Can you work these out from the model? Positions are in its coordinate system, mm. Face numbers are marked on the shaded views. A direction names the side the tool comes from. Round coordinates to 2 decimals unless told otherwise and drop trailing zeros. Order: outer loops, then holes, each group sorted by start corner. A loop starts at its lowest first (then second) coordinate and runs counter-clockwise, first axis right, second up.
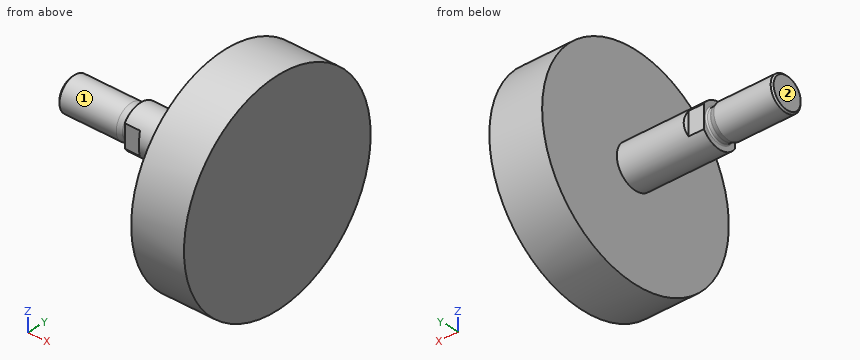
from build123d import *

# Parameters (mm, degrees)
SKETCH1_W               = 81
SKETCH1_H               = 12.5
SKETCH2_W               = 31.25
SKETCH2_H               = 62.5
CUT_EXTRUDE1_DEPTH      = 25
CUT_EXTRUDE1_DEPTH_BACK = 25


with BuildPart() as part:
    # Sketch1 → Revolve1 (revolve)
    with BuildSketch(Plane.XY):
        with Locations((29.5, 6.25)):
            Rectangle(SKETCH1_W, SKETCH1_H)
    revolve(axis=Axis((70, 0, 0), (-1, 0, 0)))

    # Sketch2 → Revolve2 (revolve)
    with BuildSketch(Plane.XY):
        with Locations((54.375, 31.25)):
            Rectangle(SKETCH2_W, SKETCH2_H)
    revolve(axis=Axis((70, 0, 0), (-1, 0, 0)))

    # Sketch3 → Revolve3 (revolve)
    with BuildSketch(Plane.XY):
        with BuildLine():
            Line((-51, 0), (-51, 9.08))
            Line((-51, 9.08), (-50.08, 10))
            Line((-50.08, 10), (-16.48485129, 10))
            Line((-16.48485129, 10), (-13.724269872, 8.995230534))
            ThreePointArc((-13.724269872, 8.995230534), (-13.597990898, 8.961394185), (-13.467754764, 8.95))
            Line((-13.467754764, 8.95), (-11.75, 8.95))
            ThreePointArc((-11.75, 8.95), (-11.219669914, 9.169669914), (-11, 9.7))
            Line((-11, 9.7), (-11, 10))
            Line((-11, 10), (-10, 10))
            Line((-10, 10), (-10, 0))
            Line((-10, 0), (-51, 0))
        make_face()
    revolve(axis=Axis((-10, 0, 0), (-1, 0, 0)))

    # Sketch4 → Cut-Extrude1 (cut, two sides)
    with BuildSketch(Plane.XY) as cut_extrude1_sk:
        Polygon((-67, -28), (8.103629711, -28), (-2, -10.5), (-11, -10.5), (-11, -15.5), (-56, -15.5), (-56, 15.5), (-11, 15.5), (-11, 10.5), (-2, 10.5), (8.103629711, 28), (-67, 28), align=None)
    extrude(amount=CUT_EXTRUDE1_DEPTH, mode=Mode.SUBTRACT)
    extrude(cut_extrude1_sk.sketch, amount=-CUT_EXTRUDE1_DEPTH_BACK, mode=Mode.SUBTRACT)


solid = part.part
(1) I want a section at D-D, the plane z = -35. List the corners of the cut face in (x, y) for me, plus the area to 3 significant figures.
(2) I want a section at B-B, the plane y = 0. List the corners of the cut face in (x, z) for me.
(3) On a 3-axis mill with a long thin cutter (end or side, diameter ignored), from which of +Z, -Z, +X, -X, +Y, -Y can I reach the whole of each face in a straight line? I mean the marked faces 1 and 2. Say none if no direction works.
(4) I want a section at A-A, the plane z = 0. List the corners of the cut face in (x, y) for me.
(5) I want a section at C-C, the plane x = 4.5. List the corners of the cut face in (y, z) for me.
(6) Please list where these lines run through material, in increasing order: probe 1 along X at (y, z) = (-4, 23.5); probe 2 along Y at (x, z) = (-31.5, 4.5); probe 3 along Z at (x, y) = (65, 0).
(7) I'm going to push flat-ended pins straight in: pin 1 Ø1.5 at (y, z) = (-44.5, -2.5) entering from -X; pin 2 Ø12 at (x, z) = (46, 9.5) entering from -Y; pin 3 Ø2.5 at (x, z) = (-8.5, 0) entering from +Y; pin 4 Ø12 at (x, y) = (-15.5, 21.5) entering from -Z. Where does each tip first touch, or does it pass through?
Ans:
1. outline: (38.75, -51.78) - (70, -51.78) - (70, 51.78) - (38.75, 51.78) - close
1. area: 3,240 mm2
2. outline: (-51, -9.08) - (-50.08, -10) - (-16.48, -10) - (-13.72, -9) arc R0.75 cw to (-13.47, -8.95) - (-11.75, -8.95) arc R0.75 cw to (-11, -9.7) - (-11, -12.5) - (38.75, -12.5) - (38.75, -62.5) - (70, -62.5) - (70, 62.5) - (38.75, 62.5) - (38.75, 12.5) - (-11, 12.5) - (-11, 9.7) arc R0.75 cw to (-11.75, 8.95) - (-13.47, 8.95) arc R0.75 cw to (-13.72, 9) - (-16.48, 10) - (-50.08, 10) - (-51, 9.08) - close
3. face 1: -X
3. face 2: +Z, -Z, -X, +Y, -Y
4. outline: (-51, -9.08) - (-50.08, -10) - (-16.48, -10) - (-13.72, -9) arc R0.75 cw to (-13.47, -8.95) - (-11.75, -8.95) arc R0.75 cw to (-11, -9.7) - (-11, -10.5) - (-2, -10.5) - (-0.85, -12.5) - (38.75, -12.5) - (38.75, -62.5) - (70, -62.5) - (70, 62.5) - (38.75, 62.5) - (38.75, 12.5) - (-0.85, 12.5) - (-2, 10.5) - (-11, 10.5) - (-11, 9.7) arc R0.75 cw to (-11.75, 8.95) - (-13.47, 8.95) arc R0.75 cw to (-13.72, 9) - (-16.48, 10) - (-50.08, 10) - (-51, 9.08) - close
5. outline: circle Ø25 at (0, 0)
6. probe 1: x = 38.75 to 70
6. probe 2: y = -8.93 to 8.93
6. probe 3: z = -62.5 to 62.5
7. pin 1: stops at x = 38.75
7. pin 2: stops at y = -62.4
7. pin 3: stops at y = 10.5
7. pin 4: passes through
